Verification items for the finished model (mm, model axes). Face numbers are marked on the shaded views. A direction names the side the tool comes from. Round coordinates to 2 decimals unless told otherwise and drop trailing zeros. Order: outer loops, then holes, each group sorted by start corner. A loop starts at its lowest first (then second) coordinate and runs counter-clockwise, first axis right, second up. Notation, with made-up numbers: (80, 32) -> (105, 32) arc R4 cw to (105, 36) -> close; hole circle Ø7 at (73.25, -10). An arc over 180 degrees is marked (long way). Answer in a Markdown table with one row per item. Add a question column.
```python
from build123d import *

# Parameters (mm, degrees)
SKETCH_1_W          = 40.2
SKETCH_1_H          = 39.8
SKETCH_1_R          = 1.75
SKETCH_1_H_2        = 3.2
EXTRUDE_1_DEPTH     = 3.2
SKETCH_2_W          = 40.2
SKETCH_2_H          = 3.2
EXTRUDE_2_DEPTH     = 43.8
SKETCH_3_R          = 1.5
CUT_EXTRUDE_1_DEPTH = 44
SKETCH_4_R          = 3.028542632
SKETCH_4_R_2        = 1.5
CUT_EXTRUDE_2_DEPTH = 1
CUT_EXTRUDE_3_DEPTH = 44


with BuildPart() as part:
    # 草图1 → 凸台-拉伸1 (new body)
    with BuildSketch(Plane.XY):
        with Locations((20.1, 23.1)):
            Rectangle(SKETCH_1_W, SKETCH_1_H)
        with Locations((5.25, 10.75)):
            Circle(SKETCH_1_R, mode=Mode.SUBTRACT)
        with Locations((35.25, 10.75)):
            Circle(SKETCH_1_R, mode=Mode.SUBTRACT)
        with Locations((5.25, 34.95)):
            Circle(SKETCH_1_R, mode=Mode.SUBTRACT)
        with Locations((35.25, 34.95)):
            Circle(SKETCH_1_R, mode=Mode.SUBTRACT)
        with Locations((20.1, 1.6)):
            Rectangle(SKETCH_1_W, SKETCH_1_H_2)
    extrude(amount=EXTRUDE_1_DEPTH)

    # 草图2 → 凸台-拉伸2 (add)
    with BuildSketch(Plane(origin=(0, 0, 0), x_dir=(-1, 0, 0), z_dir=(0, 0, -1))):
        with Locations((-20.1, 1.6)):
            Rectangle(SKETCH_2_W, SKETCH_2_H)
    extrude(amount=EXTRUDE_2_DEPTH)

    # 草图3 → 切除-拉伸1 (cut, through all)
    with BuildSketch(Plane.XZ):
        with BuildLine():
            Line((13.6, -23.8), (13.6, -30.8))
            ThreePointArc((13.6, -30.8), (20.1, -37.3), (26.6, -30.8))
            Line((26.6, -30.8), (26.6, -16.8))
            ThreePointArc((26.6, -16.8), (20.1, -10.3), (13.6, -16.8))
            Line((13.6, -16.8), (13.6, -23.8))
        make_face()
        with Locations((4.6, -23.8)):
            Circle(SKETCH_3_R)
        with Locations((12.35, -10.376606241)):
            Circle(SKETCH_3_R)
        with Locations((27.85, -10.376606241)):
            Circle(SKETCH_3_R)
        with Locations((35.6, -23.8)):
            Circle(SKETCH_3_R)
        with Locations((27.85, -37.223393759)):
            Circle(SKETCH_3_R)
        with Locations((12.35, -37.223393759)):
            Circle(SKETCH_3_R)
    extrude(amount=-CUT_EXTRUDE_1_DEPTH, mode=Mode.SUBTRACT)

    # 草图4 → 切除-拉伸2 (cut)
    with BuildSketch(Plane.XZ):
        with Locations((27.85, -37.223393759)):
            Circle(SKETCH_4_R)
        with Locations((27.85, -37.223393759)):
            Circle(SKETCH_4_R_2, mode=Mode.SUBTRACT)
        with Locations((12.35, -37.223393759)):
            Circle(SKETCH_4_R)
        with Locations((12.35, -37.223393759)):
            Circle(SKETCH_4_R_2, mode=Mode.SUBTRACT)
        with Locations((35.6, -23.8)):
            Circle(SKETCH_4_R)
        with Locations((35.6, -23.8)):
            Circle(SKETCH_4_R_2, mode=Mode.SUBTRACT)
        with Locations((27.85, -10.376606241)):
            Circle(SKETCH_4_R)
        with Locations((27.85, -10.376606241)):
            Circle(SKETCH_4_R_2, mode=Mode.SUBTRACT)
        with Locations((4.6, -23.8)):
            Circle(SKETCH_4_R)
        with Locations((12.35, -10.376606241)):
            Circle(SKETCH_4_R)
    extrude(amount=-CUT_EXTRUDE_2_DEPTH, mode=Mode.SUBTRACT)

    # 草图5 → 切除-拉伸3 (cut, through all)
    with BuildSketch(Plane.XZ):
        with BuildLine():
            ThreePointArc((18.097501561, -43.8), (5.195970031, -37.286285281), (0, -23.8))
            Line((0, -23.8), (0, -43.8))
            Line((0, -43.8), (18.097501561, -43.8))
        make_face()
        with BuildLine():
            Line((40.2, -43.8), (40.2, -23.8))
            ThreePointArc((40.2, -23.8), (35.004029969, -37.286285281), (22.102498439, -43.8))
            Line((22.102498439, -43.8), (40.2, -43.8))
        make_face()
    extrude(amount=-CUT_EXTRUDE_3_DEPTH, mode=Mode.SUBTRACT)


solid = part.part
```
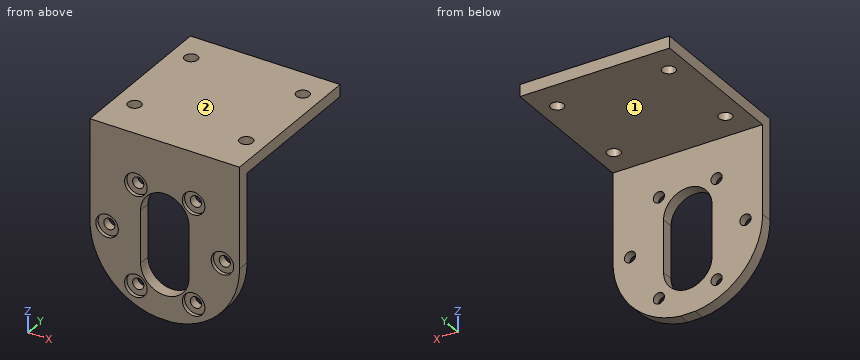
1) Cross-section at C-C, the plane x = 12.35. Record the boundary of the cut face in (y, z), and give its area (3 significant figures).
2) Tool access check on the marked faces 1 and 2. Record the directions out of +Z, -Z, +X, -X, +Y, -Y that give a thin tool (end or side, any length) a straight path to the whole face; none if there is none.
3) Thickness scan on L1, parallel to Z at x = 9, y = 12; L2, parallel to Z at x = 12.35, y = 0.25. Record the ranges inside material, lowest first. Write a range as [from, to].
4) Cross-section at D-D, the plane x = 35.25. Record the boundary of the cut face in (y, z), and give its area (3 significant figures).
5) Cross-section at A-A, the plane x = 20.1. Record the boundary of the cut face in (y, z).
6) Cross-section at B-B, the plane y = 34.95. Record the boundary of the cut face in (x, z).
7) Depth check by flat-ended pin: P1, Ø3.5, axis at x = 27.85, z = -37.22, coming from the +Y side; P2, Ø2, axis at x = 35, y = 21, coming from the -Z side; P3, Ø3, axis at x = 11, z = -10, coming from the -Y side. Enter the tip coordinate at first touch or a pass-through.
Results below:
| question | item | result |
|---|---|---|
| 1 | outline | (0, -42.35) -> (3.2, -42.35) -> (3.2, -38.72) -> (1, -38.72) -> (1, -40.25) -> (0, -40.25) -> close; (0, -34.19) -> (1, -34.19) -> (1, -35.72) -> (3.2, -35.72) -> (3.2, -11.88) -> (1, -11.88) -> (1, -13.41) -> (0, -13.41) -> close; (0, -7.35) -> (1, -7.35) -> (1, -8.88) -> (3.2, -8.88) -> (3.2, 0) -> (43, 0) -> (43, 3.2) -> (0, 3.2) -> close |
| 1 | area | 248 mm² |
| 2 | face 1 | -Z, +X, -X, +Y |
| 2 | face 2 | +Z, +X, -X, +Y, -Y |
| 3 | L1 | [0, 3.2] |
| 3 | L2 | [-42.35, -40.25], [-34.19, -13.41], [-7.35, 3.2] |
| 4 | outline | (0, -37.01) -> (3.2, -37.01) -> (3.2, -25.26) -> (1, -25.26) -> (1, -26.81) -> (0, -26.81) -> close; (0, -20.79) -> (1, -20.79) -> (1, -22.34) -> (3.2, -22.34) -> (3.2, 0) -> (9, 0) -> (9, 3.2) -> (0, 3.2) -> close; (12.5, 0) -> (33.2, 0) -> (33.2, 3.2) -> (12.5, 3.2) -> close; (36.7, 0) -> (43, 0) -> (43, 3.2) -> (36.7, 3.2) -> close |
| 4 | area | 221 mm² |
| 5 | outline | (0, -43.8) -> (3.2, -43.8) -> (3.2, -37.3) -> (0, -37.3) -> close; (0, -10.3) -> (3.2, -10.3) -> (3.2, 0) -> (43, 0) -> (43, 3.2) -> (0, 3.2) -> close |
| 6 | outline | (0, 0) -> (3.5, 0) -> (3.5, 3.2) -> (0, 3.2) -> close; (7, 0) -> (33.5, 0) -> (33.5, 3.2) -> (7, 3.2) -> close; (37, 0) -> (40.2, 0) -> (40.2, 3.2) -> (37, 3.2) -> close |
| 7 | P1 | y = 3.2 |
| 7 | P2 | z = 0 |
| 7 | P3 | y = 1 |
